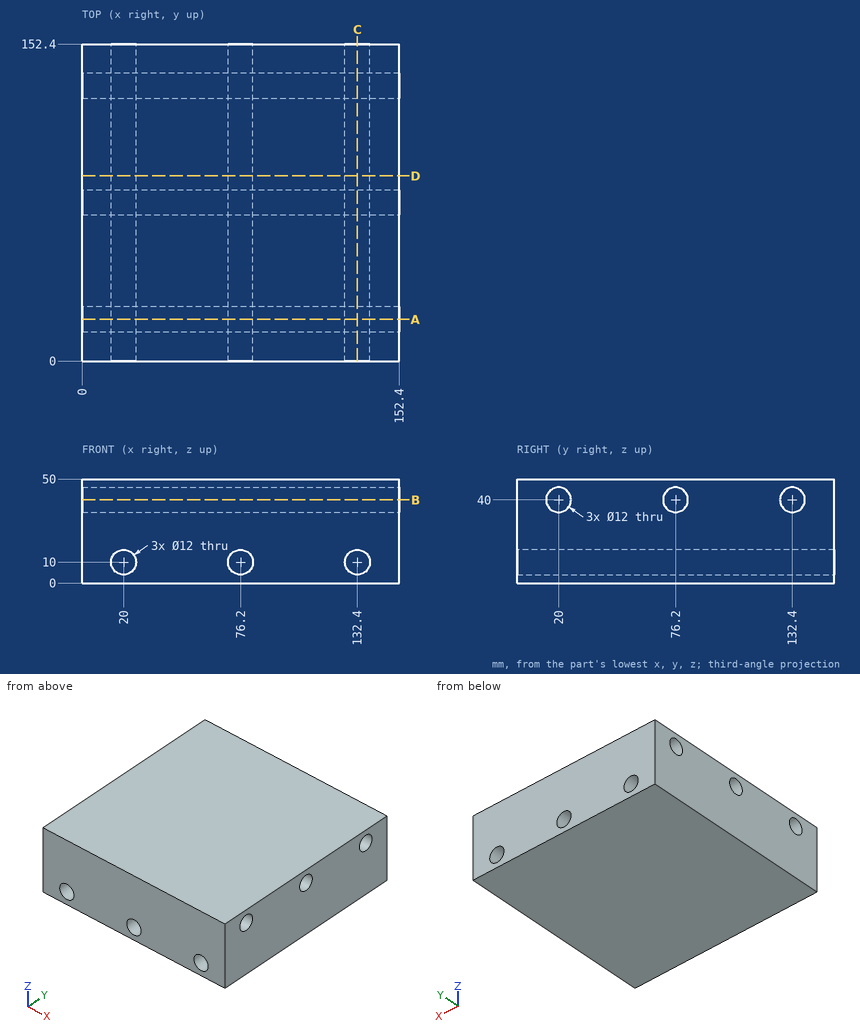
Study the drawing (mm; zero at the part's minimum x, y, z) and answer. Give positions to 0.01 mm unless a question says otherwise; leave off trailing zeros. Write each loop counter-clockwise with the first axis right and the second up, starting at its lowest first coordinate (ties: lowest second). Pieces come first, ordered by that corner, then holes. Notation, with made-up numbers: (-23.5, 58.25) -> (1.5, 58.25) arc R11 cw to (1.5, 76.25) -> close; hole circle Ø9 at (-35.75, 68.25). An arc over 180 degrees is marked (long way). Write item = value, one per line.
Q1. Section D-D on y = 89 is taken. Determine the outline of the cut face in (x, z).
Computed values:
outline = (0, 0) -> (152.4, 0) -> (152.4, 50) -> (0, 50) -> close; hole circle Ø12 at (20, 10); hole circle Ø12 at (76.2, 10); hole circle Ø12 at (132.4, 10)
Q2. A flat-ended cylindrical pin translates along its axis: pin 1 Ø10 at (x, y) = (65, 69.5) entering from -Z. Find the tip coordinate at first contact, or state that the pin passes through.
Computed values:
pin_1 = 0
Q3. Section A-A on y = 20 is taken. Determine the outline of the cut face in (x, z), and give its area (3 significant figures).
Computed values:
outline = (0, 0) -> (152.4, 0) -> (152.4, 34) -> (0, 34) -> close; (0, 46) -> (152.4, 46) -> (152.4, 50) -> (0, 50) -> close; hole circle Ø12 at (20, 10); hole circle Ø12 at (76.2, 10); hole circle Ø12 at (132.4, 10)
area = 5,450 mm^2
Q4. Consider line 1 along X through (y, z) = (94.5, 10); line 2 along Z through (x, y) = (114.5, 20); line 3 along Z through (x, y) = (132, 109). Determine where each line is inside the solid, lowest interval first.
Computed values:
line_1 = 0 to 14, 26 to 70.2, 82.2 to 126.4, 138.4 to 152.4
line_2 = 0 to 34, 46 to 50
line_3 = 0 to 4.01, 15.99 to 50
Q5. Section C-C on x = 132.4 is taken. Determine the outline of the cut face in (y, z).
Computed values:
outline = (0, 0) -> (152.4, 0) -> (152.4, 4) -> (0, 4) -> close; (0, 16) -> (152.4, 16) -> (152.4, 50) -> (0, 50) -> close; hole circle Ø12 at (20, 40); hole circle Ø12 at (76.2, 40); hole circle Ø12 at (132.4, 40)
Q6. Section B-B on z = 40 is taken. Determine the outline of the cut face in (x, y), and give its area (3 significant figures).
Computed values:
outline = (0, 0) -> (152.4, 0) -> (152.4, 14) -> (0, 14) -> close; (0, 26) -> (152.4, 26) -> (152.4, 70.2) -> (0, 70.2) -> close; (0, 82.2) -> (152.4, 82.2) -> (152.4, 126.4) -> (0, 126.4) -> close; (0, 138.4) -> (152.4, 138.4) -> (152.4, 152.4) -> (0, 152.4) -> close
area = 17,700 mm^2
